Geometry check sheet. Reference: the model listing, model coordinates, mm. A direction names the side the tool comes from. Give positions to 0.01 mm unless a question says otherwise; leave off trailing zeros. Write each loop counter-clockwise with the first axis right and the second up, starting at its lowest first coordinate (ties: lowest second). Pieces come first, ordered by that corner, then holes.
(1) Thickness scan on line 1 along Z through (x, y) = (16, -23); line 2 along X through (y, z) = (39, 61.5); line 3 along Y through (x, z) = (-64.5, 44). Record the ranges inside material, lowest first.
(2) Tool access check on faces 1 (the cylindrical face through (-18.272, 15.188, 0.986)), 2 (the flat face through (25.688, 13, 63)). Record the directions out of +Z, -Z, +X, -X, +Y, -Y that give a thin tool (end or side, any length) a straight path to the whole face; none if there is none.
(3) Cross-section at C-C (z = 22). Record the boundary of the cut face in (x, y), and give its area (3 significant figures).
(4) Cross-section at B-B (x = -63). Record the boundary of the cut face in (y, z).
(5) Depth check by flat-ended pin: P1, Ø1.5, axis at x = -56.5, z = 34.5, coming from the -Y side. Enter the tip coordinate at first touch or a pass-through.
(6) Mould release check, pull along Z, two halves, no side actions. Record for faces 3 (the flat face through (-22, 57.738, 63)), 4 (the flat face through (-22, 15, 0)), 5 (the flat face through (-70.318, 14, 63)): +Z half, -Z half, draft (parallel to the pull), parting line (faces both ways), or undercut.
(7) Cross-section at A-A (y = 35.5). Record the boundary of the cut face in (x, z), and give its area (3 significant figures).
```python
from build123d import *

# Parameters (mm, degrees)
F0_W     = 98.006491
F0_H     = 89.854028
F1_DEPTH = 127
F3_W     = 96.006491
F3_H     = 87.854028
F4_DEPTH = 84.733695
F5_T     = -2
F7_D     = 5


with BuildPart() as f1:
    # F0 (on Top) → F1 (new body)
    with BuildSketch(Plane.XY):
        with Locations((-21.314843, 14.810821)):
            Rectangle(F0_W, F0_H)
    extrude(amount=F1_DEPTH)

    # F3 (on face) → F4 (join)
    with BuildSketch(Plane.XY.offset(127)):
        with Locations((-21.314843, 14.810821)):
            Rectangle(F3_W, F3_H)
    extrude(amount=-F4_DEPTH)

    # F5
    f5_openings = [f1.faces().sort_by_distance(p)[0] for p in [
        (-21.314843, -30.116193, 63.5),
    ]]
    offset(amount=F5_T, openings=f5_openings)

    # F7 (through all)
    with Locations(Plane.XY.offset(127)):
        with Locations((-15.962919, 16.145797)):
            Hole(F7_D / 2)


solid = f1.part
```
Reply:
1. line 1: z = 0 to 2, 125 to 127
1. line 2: x = -70.32 to -68.32, 25.69 to 27.69
1. line 3: y = 57.74 to 59.74
2. face 1: +Z, -Z
2. face 2: -Y
3. outline: (-70.32, -30.12) - (-68.32, -30.12) - (-68.32, 57.74) - (25.69, 57.74) - (25.69, -30.12) - (27.69, -30.12) - (27.69, 59.74) - (-70.32, 59.74) - close
3. area: 547 mm2
4. outline: (-30.12, 0) - (59.74, 0) - (59.74, 127) - (-30.12, 127) - (-30.12, 125) - (57.74, 125) - (57.74, 2) - (-30.12, 2) - close
5. P1: stops at y = 57.74
6. face 3: undercut
6. face 4: -Z half
6. face 5: draft
7. outline: (-70.32, 0) - (27.69, 0) - (27.69, 127) - (-70.32, 127) - close; hole (-68.32, 2) - (25.69, 2) - (25.69, 125) - (-68.32, 125) - close
7. area: 884 mm2
